```python
from build123d import *

# Parameters (mm, degrees)
F1_DEPTH       = 50.8
F3_D           = 7.9248
F3_CBORE_D     = 12.7
F3_CBORE_DEPTH = 6.096
F5_DEPTH       = 134.531275
F7_DEPTH       = 118.529275


with BuildPart() as f1:
    # F0 (on Front) → F1 (new body)
    with BuildSketch(Plane.XZ):
        Polygon((0, 0), (85.852, 0), (131.70327, -45.85127), (140.683526, -36.871014), (102.60724, 1.205272), (91.112512, 12.7), (0, 12.7), align=None)
        Polygon((102.60724, 1.205272), (140.683526, -36.871014), (149.663782, -27.890758), (111.587496, 10.185528), align=None)
    extrude(amount=F1_DEPTH)

    # F3 (through all)
    with Locations(Plane(origin=(0, 0, 0), x_dir=(1, 0, 0), z_dir=(0, 0, -1))):
        with Locations((15.748, 38.1), (69.596, 38.1), (69.596, 12.7), (15.748, 12.7)):
            CounterBoreHole(F3_D / 2, F3_CBORE_D / 2, F3_CBORE_DEPTH)

    # F4 (on face) → F5 (cut, through all)
    with BuildSketch(Plane(origin=(88.77727, 0, -88.77727), x_dir=(0, 1, 0), z_dir=(0.707107, 0, -0.707107))):
        Polygon((-15.748, 86.106531), (-35.052, 86.106531), (-35.052, 80.010531), (-41.148, 80.010531), (-41.148, 73.406531), (-9.652, 73.406531), (-9.652, 80.010531), (-15.748, 80.010531), align=None)
    extrude(amount=-F5_DEPTH, mode=Mode.SUBTRACT)

    # F6 (on face) → F7 (cut, through all)
    with BuildSketch(Plane(origin=(60.886512, 0, 60.886512), x_dir=(0.707107, 0, -0.707107), z_dir=(0.707107, 0, 0.707107))):
        with BuildLine():
            ThreePointArc((119.183037, 0), (123.934026, -12.307078), (125.550019, -25.4))
            Line((125.550019, -25.4), (125.550019, 0))
            Line((125.550019, 0), (119.183037, 0))
        make_face()
        with BuildLine():
            ThreePointArc((125.550019, -25.4), (123.934026, -38.492922), (119.183037, -50.8))
            Line((119.183037, -50.8), (125.550019, -50.8))
            Line((125.550019, -50.8), (125.550019, -25.4))
        make_face()
    extrude(amount=-F7_DEPTH, mode=Mode.SUBTRACT)


solid = f1.part
```
Source: CAD feature listing. Evaluate the final solid. Frame: model axes, mm. A direction names the side the tool comes from. Give positions to 0.01 mm unless a question says otherwise; leave off trailing zeros. Order: outer loops, then holes, each group sorted by start corner. A loop starts at its lowest first (then second) coordinate and runs counter-clockwise, first axis right, second up.
(1) Pull-direction query (Z, two-part tool) for faces 1 (the face through (108.457, -25.044, -22.605)), 2 (the face through (88.4, 0, -2.2)), 3 (the face through (123, -9.652, -15)); classes: +Z half, -Z half, draft (parallel to the pull), parting line (faces both ways), or undercut.
(2) Access query for faces 4 (the face through (126.27, -12.66, -13.12)), 5 (the face through (108.2, -44.6, 6.8)), 6 (the face through (19.162, -18.054, 3.005)), 7 (the face through (128, -15.748, -11)). Directions: +Z, -Z, +X, -X, +Y, -Y. A direction counts if a zero-diameter tool reaches every point of the face in a straight line with its end or side. Return the directions, or none.
(3) Section query D-D (x = 83). Return the cut outline in (y, z), plus the area to 3 significant figures.
(4) Material intervals for line 1 along X through (y, z) = (-38, 3); line 2 along X through (y, z) = (-38, 2); line 3 along Y through (x, z) = (108.5, 2), sorted ascending.
(5) Section query B-B (x = 13.5). Return the cut outline in (y, z).
(6) Section query A-A (y = -38.1). Return the cut outline in (x, z) (1 decimal).
(7) Contact query for flat-ended pins moving along their axis: P1, Ø9, axis at x = 69.596, y = -38.1, coming from the -Z side; P2, Ø14, axis at x = 17, y = -37, coming from the -Z side; P3, Ø16.5, axis at x = 69.596, y = -38.1, coming from the +Z side; P4, Ø12, axis at y = -12, z = -7.5, coming from the -X side. Output: stop coordinate, or through.
(8) Section query C-C (z = -21.5). Return the cut outline in (x, y).
Outcome:
1. face 1: -Z half
1. face 2: draft
1. face 3: undercut
2. face 4: none
2. face 5: +Z, +Y, -Y
2. face 6: -Z
2. face 7: +Z, +X
3. outline: (-50.8, 0) - (0, 0) - (0, 12.7) - (-50.8, 12.7) - close
3. area: 645 mm2
4. line 1: x = 0 to 9.4, 22.1 to 63.25, 75.95 to 100.81, 110.15 to 118.77
4. line 2: x = 0 to 9.4, 22.1 to 63.25, 75.95 to 101.81, 111.15 to 119.77
4. line 3: y = -50.8 to -41.15, -9.65 to 0
5. outline: (-50.8, 0) - (-44.04, 0) - (-44.04, 6.1) - (-41.36, 6.1) - (-41.36, 12.7) - (-50.8, 12.7) - close; (-34.84, 6.1) - (-32.16, 6.1) - (-32.16, 0) - (-18.64, 0) - (-18.64, 6.1) - (-15.96, 6.1) - (-15.96, 12.7) - (-34.84, 12.7) - close; (-9.44, 6.1) - (-6.76, 6.1) - (-6.76, 0) - (0, 0) - (0, 12.7) - (-9.44, 12.7) - close
6. outline: (0, 0) - (9.4, 0) - (9.4, 6.1) - (11.8, 6.1) - (11.8, 12.7) - (0, 12.7) - close; (19.7, 6.1) - (22.1, 6.1) - (22.1, 0) - (63.2, 0) - (63.2, 6.1) - (65.6, 6.1) - (65.6, 12.7) - (19.7, 12.7) - close; (73.6, 6.1) - (75.9, 6.1) - (75.9, 0) - (85.9, 0) - (130.6, -44.8) - (139.6, -35.8) - (91.1, 12.7) - (73.6, 12.7) - close; (107.3, 5.9) - (144.3, -31.1) - (148.6, -26.8) - (111.6, 10.2) - close
7. P1: stops at z = 6.1
7. P2: stops at z = 0
7. P3: stops at z = 12.7
7. P4: stops at x = 87.35
8. outline: (107.35, -50.8) - (143.27, -50.8) - (143.27, -35.05) - (134.65, -35.05) - (134.65, -41.15) - (125.31, -41.15) - (125.31, -9.65) - (134.65, -9.65) - (134.65, -15.75) - (143.27, -15.75) - (143.27, 0) - (107.35, 0) - close
